```python
from build123d import *

# Parameters (mm, degrees)
BOSS_EXTRU_1_DEPTH                            = 8
TROU_POUR_TARAUDAGE_POUR_TROU_TARAUD_M3_D     = 2.5
TROU_POUR_TARAUDAGE_POUR_TROU_TARAUD_M3_DEPTH = 8


with BuildPart() as part:
    # Esquisse1 → Boss.-Extru.1 (new body)
    with BuildSketch(Plane.XY):
        Polygon((2.5, -1.443375673), (2.5, 1.443375673), (0, 2.886751346), (-2.5, 1.443375673), (-2.5, -1.443375673), (0, -2.886751346), align=None)
    extrude(amount=BOSS_EXTRU_1_DEPTH)

    # Trou pour taraudage pour trou taraudé M31
    with Locations(Plane.XY.offset(8)):
        with Locations((0, 0)):
            Hole(TROU_POUR_TARAUDAGE_POUR_TROU_TARAUD_M3_D / 2, depth=TROU_POUR_TARAUDAGE_POUR_TROU_TARAUD_M3_DEPTH)


solid = part.part
```
The listing builds one solid part. Answer for the finished solid, in the listing's coordinates (mm). Give positions to 0.01 mm unless a question says otherwise; leave off trailing zeros. Loops run counter-clockwise (first coordinate to the right, second up) from the corner with the lowest first, then second, coordinate; pieces in that order, holes last. Notation, with made-up numbers: (42.5, 17.5) - (100.5, 17.5) arc R9 ccw to (100.5, 22.5) - close; hole circle Ø5 at (71, 24.5). An arc over 180 degrees is marked (long way). Return JSON: item names as keys, results as strings. Group by question number.
1. Determine the mould class of faces 1 (the flat face through (1.267, 2.155, 3.944)), 2 (the flat face through (1.233, -2.175, 3.944)), 3 (the cylindrical face through (0.27, -1.22, 3.94)) for opening direction Y: pulls with the +Y half, pulls with the -Y half, needs draft (parallel to the pull), parting line crosses it, or undercut.
2. Given pin 1 Ø2 at (x, z) = (-0.5, 2.5) entering from +Y; pin 2 Ø1 at (x, z) = (-2, 3) entering from +Y, each flat-ended and moving along its own axis, determine where each tip first touches the part or whether it passes through.
3. Find section B-B (z = 1.25). Write down the section's boundary in (x, y).
4. Find section C-C (x = -0.6). Write down the section's boundary in (y, z), then the cut area to 3 significant figures.
5. Straight lines are drawn through the part: line 1 (Y direction, x = 0.6, z = 3.75); line 2 (X direction, y = -0.85, z = 3.25); line 3 (Y direction, x = -0.1, z = 0.5). For each, find the intervals that lie inside material, in ascending order. Write a range as [from, to].
6. Find section A-A (y = 0). Write down the section's boundary in (x, z).
7. Find section D-D (y = 2.05). Write down the section's boundary in (x, z).
Verdict:
{
 "1": {"face 1": "pulls with the +Y half", "face 2": "pulls with the -Y half", "face 3": "undercut"},
 "2": {"pin 1": "stops at y = 2.89", "pin 2": "stops at y = 2.02"},
 "3": {"outline": "(-2.5, -1.44) - (0, -2.89) - (2.5, -1.44) - (2.5, 1.44) - (0, 2.89) - (-2.5, 1.44) - close; hole circle Ø2.5 at (0, 0)"},
 "4": {"outline": "(-2.54, 0) - (-1.1, 0) - (-1.1, 8) - (-2.54, 8) - close; (1.1, 0) - (2.54, 0) - (2.54, 8) - (1.1, 8) - close", "area": "23.1 mm^2"},
 "5": {"line 1": "y = [-2.54, -1.1], [1.1, 2.54]", "line 2": "x = [-2.5, -0.92], [0.92, 2.5]", "line 3": "y = [-2.83, -1.25], [1.25, 2.83]"},
 "6": {"outline": "(-2.5, 0) - (-1.25, 0) - (-1.25, 8) - (-2.5, 8) - close; (1.25, 0) - (2.5, 0) - (2.5, 8) - (1.25, 8) - close"},
 "7": {"outline": "(-1.45, 0) - (1.45, 0) - (1.45, 8) - (-1.45, 8) - close"}
}
